from build123d import *

# Parameters (mm, degrees)
F0_W     = 42
F0_H     = 60
F0_R     = 2
F1_DEPTH = 8
F3_DEPTH = 8


with BuildPart() as f1:
    # F0 (on Top) → F1 (new body)
    with BuildSketch(Plane.XY):
        Rectangle(F0_W, F0_H)
        with Locations((-16, -23)):
            Circle(F0_R, mode=Mode.SUBTRACT)
        with Locations((16, -23)):
            Circle(F0_R, mode=Mode.SUBTRACT)
        with Locations((-16, 23)):
            Circle(F0_R, mode=Mode.SUBTRACT)
        with Locations((16, 23)):
            Circle(F0_R, mode=Mode.SUBTRACT)
    extrude(amount=F1_DEPTH)

    # F2 (on face) → F3 (join)
    with BuildSketch(Plane.XY.offset(8)):
        Polygon((-13.5, 37.5), (-21, 30), (21, 30), (13.5, 37.5), align=None)
    extrude(amount=-F3_DEPTH)


solid = f1.part
Build history of the part. All positions in model axes, mm. Give positions to 0.01 mm unless a question says otherwise; leave off trailing zeros. Loops run counter-clockwise (first coordinate to the right, second up) from the corner with the lowest first, then second, coordinate; pieces in that order, holes last. Notation, with made-up numbers: (4, 31.25) -> (15, 31.25) arc R22 cw to (15, 54.25) -> close; hole circle Ø2 at (43.5, 72.25). An arc over 180 degrees is marked (long way). Answer in a Markdown table with one row per item.
Item 1: Mould opens along X. For faces 1 (the flat face through (17, 34, 4)), 2 (the cylindrical face through (-17.6, 21.8, 3.9)), 3 (the cylindrical face through (14.526, -21.648, 3.944)), 4 (the flat face through (-21, 0, 4)) say: pulls with the +X half, pulls with the -X half, needs draft (parallel to the pull), parting line crosses it, or undercut.
Findings below:
| item | result |
|---|---|
| face 1 | pulls with the +X half |
| face 2 | undercut |
| face 3 | undercut |
| face 4 | pulls with the -X half |
Item 2: Slice it at C-C on z = 7. Write the cut outline in (x, y), plus the area to 3 significant figures.
Findings below:
| item | result |
|---|---|
| outline | (-21, -30) -> (21, -30) -> (21, 30) -> (13.5, 37.5) -> (-13.5, 37.5) -> (-21, 30) -> close; hole circle Ø4 at (-16, -23); hole circle Ø4 at (-16, 23); hole circle Ø4 at (16, -23); hole circle Ø4 at (16, 23) |
| area | 2,730 mm² |
Item 3: Slice it at B-B on x = 16. Write the cut outline in (y, z).
Findings below:
| item | result |
|---|---|
| outline | (-30, 0) -> (-25, 0) -> (-25, 8) -> (-30, 8) -> close; (-21, 0) -> (21, 0) -> (21, 8) -> (-21, 8) -> close; (25, 0) -> (35, 0) -> (35, 8) -> (25, 8) -> close |
Item 4: Slice it at D-D on y = 32. Write the cut outline in (x, z).
Findings below:
| item | result |
|---|---|
| outline | (-19, 0) -> (19, 0) -> (19, 8) -> (-19, 8) -> close |
Item 5: Probe line 1 along Y through (x, z) = (-14.5, 7.75); line 2 along Y through (x, z) = (-17.5, 6.5); line 3 along Y through (x, z) = (18.5, 1.25). List the from-to ranges inside material, lowest first. Write a range as [from, to].
Findings below:
| item | result |
|---|---|
| line 1 | y = [-30, -24.32], [-21.68, 21.68], [24.32, 36.5] |
| line 2 | y = [-30, -24.32], [-21.68, 21.68], [24.32, 33.5] |
| line 3 | y = [-30, 32.5] |
Item 6: Slice it at A-A on y = -23. Write the cut outline in (x, z), plus the area to 3 significant figures.
Findings below:
| item | result |
|---|---|
| outline | (-21, 0) -> (-18, 0) -> (-18, 8) -> (-21, 8) -> close; (-14, 0) -> (14, 0) -> (14, 8) -> (-14, 8) -> close; (18, 0) -> (21, 0) -> (21, 8) -> (18, 8) -> close |
| area | 272 mm² |
Item 7: Flat gauge pin, fed straight in: P1, Ø2.5, axis at x = 16, y = 23, coming from the +Z side. Where does the tip first touch, or does it go through?
Findings below:
| item | result |
|---|---|
| P1 | passes through |
